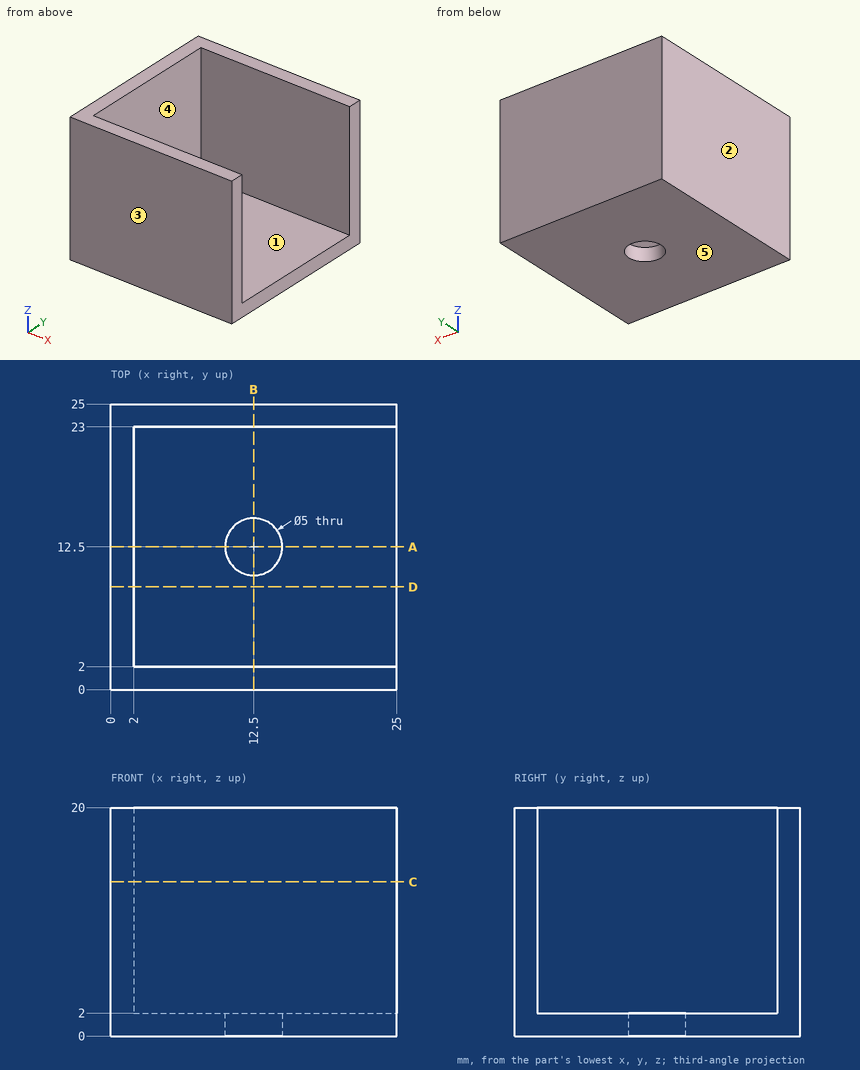
Print and shaded views of the part. All mm, measured from the part's lowest x, y and z. A direction names the side the tool comes from. Coordinates: 2 decimals unless noted, no trailing zeros. Order: outer loops, then holes, each group sorted by start corner. A loop starts at its lowest first (then second) coordinate and runs counter-clockwise, first axis right, second up. Notation, with made-up numbers: M 6,-4 L 51,-4 A12 ccw 51,8 Z; hole C 42,18.25 d7. An arc over 180 degrees is marked long. Answer as CSV lines item,"result".
1) Cut at C-C (z = 13.5). List the corners of the cut face in (x, y), then the cut area to 3 significant figures.
Verdict:
outline,"M 0,0 L 25,0 L 25,2 L 2,2 L 2,23 L 25,23 L 25,25 L 0,25 Z"
area,"142 mm2"
2) Flat gauge pins, fed straight in: P1, Ø10.5, axis at x = 13, y = 11, coming from the +Z side; P2, Ø5.5, axis at y = 12.5, z = 7.5, coming from the +X side. Where does each tip first touch, or does it go through?
Verdict:
P1,"z = 2"
P2,"x = 2"
3) 3-axis set-ups, long thin cutter, end or side, ignore diameter. For the marked faces 4 and 5: which of +Z, -Z, +X, -X, +Y, -Y reach the whole face in a straight line?
Verdict:
face 4,"+Z, +X"
face 5,"-Z, +X, -X, +Y, -Y"
4) Cut at A-A (y = 12.5). List the corners of the cut face in (x, z).
Verdict:
outline,"M 0,0 L 10,0 L 10,2 L 2,2 L 2,20 L 0,20 Z; M 15,0 L 25,0 L 25,2 L 15,2 Z"
5) Mould opens along Y. For the marked faces 1, 2 and 3 say: released by +Y, released by -Y, zero draft, split by the parting line, or undercut.
Verdict:
face 1,"undercut"
face 2,"zero draft"
face 3,"released by -Y"
6) Cut at D-D (y = 9). List the corners of the cut face in (x, z).
Verdict:
outline,"M 0,0 L 25,0 L 25,2 L 2,2 L 2,20 L 0,20 Z"
7) Cut at B-B (x = 12.5). List the corners of the cut face in (y, z), then the cut area to 3 significant figures.
Verdict:
outline,"M 0,0 L 10,0 L 10,2 L 2,2 L 2,20 L 0,20 Z; M 15,0 L 25,0 L 25,20 L 23,20 L 23,2 L 15,2 Z"
area,"112 mm2"
8) Drill centre lines: L1, parallel to Y at x = 12.5, z = 1.2; L2, parallel to Y at x = 11.5, z = 17.5; L3, parallel to Z at x = 14.75, y = 9. Where is each one in solid material? Low to high. Write a range as from..to.
Verdict:
L1,"0..10, 15..25"
L2,"0..2, 23..25"
L3,"0..2"
